from build123d import *

# Parameters (mm, degrees)
SALIENTE_EXTRUIR1_DEPTH   = 7
SALIENTE_EXTRUIR1_2_DEPTH = 7
CROQUIS2_W                = 27
CROQUIS2_H                = 51
SALIENTE_EXTRUIR2_DEPTH   = 5
CORTAR_EXTRUIR1_REACH     = 48.062
CROQUIS4_R                = 1.75
CORTAR_EXTRUIR2_DEPTH     = 5
CORTAR_EXTRUIR3_REACH     = 46.821
CROQUIS5_R                = 1.75
REDONDEO1_R               = 13
CROQUIS6_W                = 40
CROQUIS6_H                = 20
CROQUIS6_W_2              = 30
CROQUIS6_H_2              = 5.5
SALIENTE_EXTRUIR3_DEPTH   = 5
REDONDEO5_R               = 3
CORTAR_EXTRUIR4_REACH     = 46.821
CROQUIS7_W                = 10
CROQUIS7_H                = 7
CORTAR_EXTRUIR5_REACH     = 58.58
CROQUIS8_W                = 10
CROQUIS8_H                = 7
CORTAR_EXTRUIR6_REACH     = 60.108
CROQUIS10_W               = 5
CROQUIS10_H               = 9
SALIENTE_EXTRUIR4_DEPTH   = 40
CORTAR_EXTRUIR7_REACH     = 60.108
CROQUIS11_W               = 35
CROQUIS11_H               = 3.5
CORTAR_EXTRUIR8_REACH     = 60.108
CROQUIS12_R               = 3


with BuildPart() as part:
    # Croquis1 → Saliente-Extruir1 (new body)
    with BuildSketch(Plane.XY):
        Polygon((0, 0), (-22.9496732, 13.25), (-25.4496732, 8.919872981), (-2.5, -4.330127019), align=None)
    extrude(amount=SALIENTE_EXTRUIR1_DEPTH)



with BuildPart() as body_2:
    # Croquis1 → Saliente-Extruir1 2 (new body)
    with BuildSketch(Plane.XY):
        Polygon((-25.4496732, -33.330127019), (-2.5, -20.080127019), (0, -24.410254038), (-22.9496732, -37.660254038), align=None)
    extrude(amount=SALIENTE_EXTRUIR1_2_DEPTH)


with BuildPart() as part_1:
    add(part.part)

    add(body_2.part)  # Saliente-Extruir2 merges body 2
    # Croquis2 → Saliente-Extruir2 (add)
    with BuildSketch(Plane.XY.offset(7)):
        with Locations((-11.9496732, -12.25)):
            Rectangle(CROQUIS2_W, CROQUIS2_H)
    extrude(amount=SALIENTE_EXTRUIR2_DEPTH)

    # Croquis3 → Cortar-Extruir1 (cut, up to next)
    with BuildSketch(Plane(origin=(0, 0, 7), x_dir=(-1, 0, 0), z_dir=(0, 0, -1)), mode=Mode.PRIVATE) as cortar_extruir1_sk1:
        with BuildLine():
            Line((13.571492094, 0.794872981), (16.671492094, 0.794872981))
            Line((16.671492094, 0.794872981), (17.671492094, 0.794872981))
            ThreePointArc((17.671492094, 0.794872981), (23.221592496, -12.205127019), (17.671492094, -25.205127019))
            Line((17.671492094, -25.205127019), (16.671492094, -25.205127019))
            Line((16.671492094, -25.205127019), (13.571492094, -25.205127019))
            Line((13.571492094, -25.205127019), (12.571492094, -25.205127019))
            ThreePointArc((12.571492094, -25.205127019), (17.909045513, -12.205127019), (12.571492094, 0.794872981))
            Line((12.571492094, 0.794872981), (13.571492094, 0.794872981))
        make_face()
    cortar_extruir1_tool1 = extrude(cortar_extruir1_sk1.sketch, amount=-CORTAR_EXTRUIR1_REACH, mode=Mode.PRIVATE) & part_1.part
    add(cortar_extruir1_tool1.solids().sort_by_distance((-18.892381, -12.205127, 7))[0], mode=Mode.SUBTRACT)

    # Croquis4 → Cortar-Extruir2 (cut)
    with BuildSketch(Plane(origin=(-2.5, -4.330127019, 0), x_dir=(0.8660254037844369, -0.5000000000000031, 0), z_dir=(-0.500000000000003, -0.8660254037844368, 0))):
        with Locations((-22.5, 3)):
            Circle(CROQUIS4_R)
        with Locations((-4, 3)):
            Circle(CROQUIS4_R)
    extrude(amount=-CORTAR_EXTRUIR2_DEPTH, mode=Mode.SUBTRACT)

    # Croquis5 → Cortar-Extruir3 (cut, up to next)
    with BuildSketch(Plane(origin=(8.069950055, -13.977563509, 0), x_dir=(0.8660254037844367, 0.5000000000000033, 0), z_dir=(-0.5000000000000033, 0.8660254037844367, 0)), mode=Mode.PRIVATE) as cortar_extruir3_sk1:
        with Locations(Location((-34.705127019, -3, 0), (0, 0, 180))):
            Circle(CROQUIS5_R)
    cortar_extruir3_tool1 = extrude(cortar_extruir3_sk1.sketch, amount=-CORTAR_EXTRUIR3_REACH, mode=Mode.PRIVATE) & part_1.part
    # Croquis5 → Cortar-Extruir3 (cut, up to next)
    with BuildSketch(Plane(origin=(8.069950055, -13.977563509, 0), x_dir=(0.8660254037844367, 0.5000000000000033, 0), z_dir=(-0.5000000000000033, 0.8660254037844367, 0)), mode=Mode.PRIVATE) as cortar_extruir3_sk2:
        with Locations(Location((-16.205127019, -3, 0), (0, 0, 180))):
            Circle(CROQUIS5_R)
    cortar_extruir3_tool2 = extrude(cortar_extruir3_sk2.sketch, amount=-CORTAR_EXTRUIR3_REACH, mode=Mode.PRIVATE) & part_1.part
    add(cortar_extruir3_tool1.solids().sort_by_distance((-21.985572, -31.330127, 3))[0], mode=Mode.SUBTRACT)
    add(cortar_extruir3_tool2.solids().sort_by_distance((-5.964102, -22.080127, 3))[0], mode=Mode.SUBTRACT)

    # Redondeo1
    redondeo1_edges = [part_1.edges().sort_by_distance(p)[0] for p in [
        (1.5503268, 13.25, 9.5),
    ]]
    fillet(redondeo1_edges, radius=REDONDEO1_R)

    # Croquis6 → Saliente-Extruir3 (add)
    with BuildSketch(Plane.XZ.offset(37.75)):
        with Locations((21.5503268, 2)):
            Rectangle(CROQUIS6_W, CROQUIS6_H)
        with Locations((21.5503268, -1.25)):
            Rectangle(CROQUIS6_W_2, CROQUIS6_H_2, mode=Mode.SUBTRACT)
    extrude(amount=-SALIENTE_EXTRUIR3_DEPTH)

    # Redondeo5
    redondeo5_edges = [part_1.edges().sort_by_distance(p)[0] for p in [
        (1.5503268, -35.25, 7),
    ]]
    fillet(redondeo5_edges, radius=REDONDEO5_R)

    # Croquis7 → Cortar-Extruir4 (cut, up to next)
    with BuildSketch(Plane(origin=(8.069950055, -13.977563509, 0), x_dir=(0.8660254037844367, 0.5000000000000033, 0), z_dir=(-0.5000000000000033, 0.8660254037844367, 0)), mode=Mode.PRIVATE) as cortar_extruir4_sk1:
        with Locations((-25.455127019, -3.5)):
            Rectangle(CROQUIS7_W, CROQUIS7_H)
    cortar_extruir4_tool1 = extrude(cortar_extruir4_sk1.sketch, amount=-CORTAR_EXTRUIR4_REACH, mode=Mode.PRIVATE) & part_1.part
    add(cortar_extruir4_tool1.solids().sort_by_distance((-13.974837, -26.705127, 3.5))[0], mode=Mode.SUBTRACT)

    # Croquis8 → Cortar-Extruir5 (cut, up to next)
    with BuildSketch(Plane(origin=(-2.5, -4.330127019, 0), x_dir=(0.8660254037844369, -0.5000000000000031, 0), z_dir=(-0.500000000000003, -0.8660254037844368, 0)), mode=Mode.PRIVATE) as cortar_extruir5_sk1:
        with Locations((-13.25, 3.5)):
            Rectangle(CROQUIS8_W, CROQUIS8_H)
    cortar_extruir5_tool1 = extrude(cortar_extruir5_sk1.sketch, amount=-CORTAR_EXTRUIR5_REACH, mode=Mode.PRIVATE) & part_1.part
    add(cortar_extruir5_tool1.solids().sort_by_distance((-13.974837, 2.294873, 3.5))[0], mode=Mode.SUBTRACT)

    # Croquis9 → Cortar-Extruir6 (cut, up to next)
    with BuildSketch(Plane(origin=(0, 0, 7), x_dir=(-1, 0, 0), z_dir=(0, 0, -1)), mode=Mode.PRIVATE) as cortar_extruir6_sk1:
        with BuildLine():
            Line((25.4496732, -3.205127019), (25.4496732, -21.205127019))
            Line((25.4496732, -21.205127019), (20.619740445, -21.526985187))
            ThreePointArc((20.619740445, -21.526985187), (23.220621564, -12.392083108), (20.810049764, -3.205127019))
            Line((20.810049764, -3.205127019), (25.4496732, -3.205127019))
        make_face()
    cortar_extruir6_tool1 = extrude(cortar_extruir6_sk1.sketch, amount=-CORTAR_EXTRUIR6_REACH, mode=Mode.PRIVATE) & part_1.part
    add(cortar_extruir6_tool1.solids().sort_by_distance((-23.839782, -12.328925, 7))[0], mode=Mode.SUBTRACT)

    # Croquis10 → Saliente-Extruir4 (add)
    with BuildSketch(Plane(origin=(1.5503268, 0, 0), x_dir=(0, 0, -1), z_dir=(1, 0, 0))):
        with Locations((-9.5, -28.25)):
            Rectangle(CROQUIS10_W, CROQUIS10_H)
    extrude(amount=SALIENTE_EXTRUIR4_DEPTH)

    # Croquis11 → Cortar-Extruir7 (cut, up to next)
    with BuildSketch(Plane(origin=(0, 0, 7), x_dir=(-1, 0, 0), z_dir=(0, 0, -1)), mode=Mode.PRIVATE) as cortar_extruir7_sk1:
        with Locations((-19.0503268, -28.25)):
            Rectangle(CROQUIS11_W, CROQUIS11_H)
    cortar_extruir7_tool1 = extrude(cortar_extruir7_sk1.sketch, amount=-CORTAR_EXTRUIR7_REACH, mode=Mode.PRIVATE) & part_1.part
    add(cortar_extruir7_tool1.solids().sort_by_distance((19.050327, -28.25, 7))[0], mode=Mode.SUBTRACT)

    # Croquis12 → Cortar-Extruir8 (cut, up to next)
    with BuildSketch(Plane(origin=(0, 0, 7), x_dir=(-1, 0, 0), z_dir=(0, 0, -1)), mode=Mode.PRIVATE) as cortar_extruir8_sk1:
        with Locations((10.4496732, -32.75)):
            Circle(CROQUIS12_R)
    cortar_extruir8_tool1 = extrude(cortar_extruir8_sk1.sketch, amount=-CORTAR_EXTRUIR8_REACH, mode=Mode.PRIVATE) & part_1.part
    # Croquis12 → Cortar-Extruir8 (cut, up to next)
    with BuildSketch(Plane(origin=(0, 0, 7), x_dir=(-1, 0, 0), z_dir=(0, 0, -1)), mode=Mode.PRIVATE) as cortar_extruir8_sk2:
        with Locations(Location((9.4496732, 8.25, 0), (0, 0, 180))):
            Circle(CROQUIS12_R)
    cortar_extruir8_tool2 = extrude(cortar_extruir8_sk2.sketch, amount=-CORTAR_EXTRUIR8_REACH, mode=Mode.PRIVATE) & part_1.part
    add(cortar_extruir8_tool1.solids().sort_by_distance((-10.449673, -32.75, 7))[0], mode=Mode.SUBTRACT)
    add(cortar_extruir8_tool2.solids().sort_by_distance((-9.449673, 8.25, 7))[0], mode=Mode.SUBTRACT)


solid = part_1.part
Geometry check sheet. Reference: the model listing, model coordinates, mm. A direction names the side the tool comes from. Round coordinates to 2 decimals unless told otherwise and drop trailing zeros. Loops run counter-clockwise (first coordinate to the right, second up) from the corner with the lowest first, then second, coordinate; pieces in that order, holes last. Notation, with made-up numbers: (44, 2) -> (55, 2) arc R27 cw to (55, 35) -> close; hole circle Ø7 at (24.5, 83.5). An arc over 180 degrees is marked (long way). Answer as a JSON object with one key per item and string values. Group by question number.
Item 1: Set-up check for faces 1 (the face through (-23.069, -21.364, 9.465)), 2 (the face through (-17.07, 6.93, 3.45)), 3 (the face through (-21.93, 6.89, 5.01)), 4 (the face through (-8.41, -26.34, 3.55)): record each of +Z, -Z, +X, -X, +Y, -Y from which the full face is reachable in a straight line by a thin tool's end or side.
Item 2: Cross-section at A-A, the plane x = 3. Record the cut outline in (y, z), plus the area to 4 significant figures.
Item 3: Cross-section at B-B, the plane z = 8.5. Record the cut outline in (x, y), plus the area to 3 significant figures.
Item 4: Release check for a two-part mould opening along Y. For faces 5 (the face through (-6.12, -2.24, 5.01)), 6 (the face through (-2.359, 9.543, 9.535)), 7 (the face through (-25.45, 5, 9)), 8 (the face through (-19.287, -23.437, 9.465)) record: pulls with the +Y half, pulls with the -Y half, needs draft (parallel to the pull), parting line crosses it, or undercut.
Item 5: Cross-section at C-C, the plane z = -2.25. Record the cut outline in (x, y).
Item 6: Depth check by flat-ended pin: pin 1 Ø4 at (y, z) = (-19.5, -1) entering from +X; pin 2 Ø5.5 at (x, y) = (-9.45, 8.25) entering from +Z; pin 3 Ø12 at (x, z) = (29.5, 6) entering from +Y; pin 4 Ø2.5 at (x, y) = (-22, -33.5) entering from -Z. Enter the tip coordinate at first touch or a pass-through.
Item 7: Thickness scan on line 1 along Y through (x, z) = (16, 9.5); line 2 along X through (y, z) = (-33.5, -1.25); line 3 along Z through (x, y) = (-14, -34.5). Record the ranges inside material, lowest first.
Determined:
{
 "1": {"face 1": "+Z, -Z", "face 2": "-Z, +X", "face 3": "-Z, -X", "face 4": "-Z, -X, -Y"},
 "2": {"outline": "(-37.75, -8) -> (-32.75, -8) -> (-32.75, 7) -> (-30, 7) -> (-30, 12) -> (-37.75, 12) -> close; (-26.5, 7) -> (-23.75, 7) -> (-23.75, 12) -> (-26.5, 12) -> close", "area": "127.5 mm²"},
 "3": {"outline": "(-25.45, -37.75) -> (41.55, -37.75) -> (41.55, -23.75) -> (1.55, -23.75) -> (1.55, 0.25) arc R13 ccw to (-11.45, 13.25) -> (-25.45, 13.25) -> (-25.45, -3.21) -> (-20.81, -3.21) arc R18 cw to (-17.67, 0.79) -> (-12.57, 0.79) arc R18.5 ccw to (-12.57, -25.21) -> (-17.67, -25.21) arc R18 cw to (-20.62, -21.53) -> (-25.45, -21.21) -> close; hole circle Ø6 at (-10.45, -32.75); hole circle Ø6 at (-9.45, 8.25); hole (1.55, -30) -> (36.55, -30) -> (36.55, -26.5) -> (1.55, -26.5) -> close", "area": "1,530 mm²"},
 "4": {"face 5": "undercut", "face 6": "pulls with the +Y half", "face 7": "needs draft", "face 8": "undercut"},
 "5": {"outline": "(1.55, -37.75) -> (6.55, -37.75) -> (6.55, -32.75) -> (1.55, -32.75) -> close; (36.55, -37.75) -> (41.55, -37.75) -> (41.55, -32.75) -> (36.55, -32.75) -> close"},
 "6": {"pin 1": "stops at x = -1.83", "pin 2": "passes through", "pin 3": "stops at y = -23.75", "pin 4": "stops at z = 0"},
 "7": {"line 1": "y = -37.75 to -30, -26.5 to -23.75", "line 2": "x = 1.55 to 6.55, 36.55 to 41.55", "line 3": "z = 7 to 12"}
}
